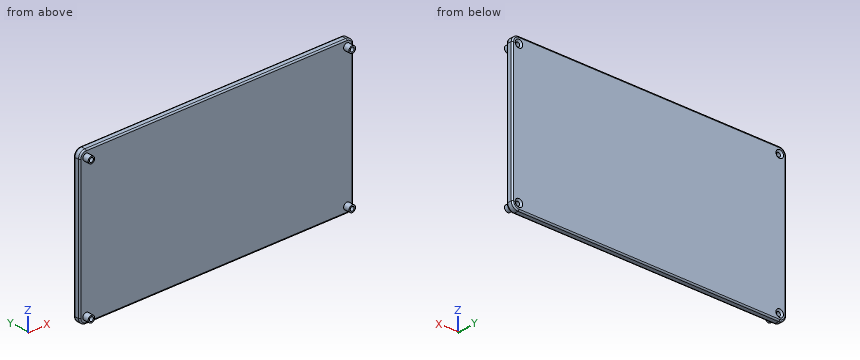
```python
from build123d import *

# Parameters (mm, degrees)
SKETCH1_W                                         = 210
SKETCH1_H                                         = 113
BOSS_EXTRUDE1_DEPTH                               = 5
FILLET1_R                                         = 5
FILLET2_R                                         = 1
CSK_FOR_4_FLAT_HEAD_MACHINE_SCREW_100_D           = 2.9464
CSK_FOR_4_FLAT_HEAD_MACHINE_SCREW_100_CSINK_D     = 5.715
CSK_FOR_4_FLAT_HEAD_MACHINE_SCREW_100_CSINK_ANGLE = 100
SKETCH8_R                                         = 2.4732
BOSS_EXTRUDE2_DEPTH                               = 4.525
SKETCH10_R                                        = 1.525
CUT_EXTRUDE1_DEPTH                                = 1
CUT_EXTRUDE1_DEPTH_BACK                           = 10.525
SKETCH11_R                                        = 2.525
BOSS_EXTRUDE3_DEPTH                               = 4.525
SKETCH14_R                                        = 1.525
CUT_EXTRUDE2_DEPTH                                = 10.5250001
SKETCH15_R                                        = 2.525
BOSS_EXTRUDE6_DEPTH                               = 4.525
SKETCH16_R                                        = 1.525
CUT_EXTRUDE3_DEPTH                                = 10.5250001
SKETCH17_R                                        = 2.525
BOSS_EXTRUDE7_DEPTH                               = 4.525
SKETCH18_R                                        = 1.525
CUT_EXTRUDE4_DEPTH                                = 10.5250001


with BuildPart() as part:
    # Sketch1 → Boss-Extrude1 (new body)
    with BuildSketch(Plane(origin=(0, 0, 0), x_dir=(1, 0, 0), z_dir=(0, 1, 0))):
        Rectangle(SKETCH1_W, SKETCH1_H)
    extrude(amount=BOSS_EXTRUDE1_DEPTH)

    # Fillet1
    fillet1_edges = [part.edges().sort_by_distance(p)[0] for p in [
        (105, 2.5, 56.5),
        (-105, 2.5, 56.5),
        (-105, 2.5, -56.5),
        (105, 2.5, -56.5),
    ]]
    fillet(fillet1_edges, radius=FILLET1_R)

    # Fillet2
    fillet2_edges = [part.edges().sort_by_distance(p)[0] for p in [
        (-105, 0, 0),
        (-105, 5, 0),
        (105, 0, 0),
        (0, 0, 56.5),
        (0, 0, -56.5),
        (103.535533906, 0, -55.035533906),
        (103.535533906, 0, 55.035533906),
        (-103.535533906, 0, 55.035533906),
        (-103.535533906, 0, -55.035533906),
        (0, 5, -56.5),
        (105, 5, 0),
        (0, 5, 56.5),
        (103.535533906, 5, -55.035533906),
        (103.535533906, 5, 55.035533906),
        (-103.535533906, 5, 55.035533906),
        (-103.535533906, 5, -55.035533906),
    ]]
    fillet(fillet2_edges, radius=FILLET2_R)

    # CSK for #4 Flat Head Machine Screw (100)1 (through all)
    with Locations(Plane(origin=(0, 5, 0), x_dir=(1, 0, 0), z_dir=(0, 1, 0))):
        with Locations((-100, -51.5), (100, 51.5), (100, -51.5), (-100, 51.5)):
            CounterSinkHole(CSK_FOR_4_FLAT_HEAD_MACHINE_SCREW_100_D / 2, CSK_FOR_4_FLAT_HEAD_MACHINE_SCREW_100_CSINK_D / 2, counter_sink_angle=CSK_FOR_4_FLAT_HEAD_MACHINE_SCREW_100_CSINK_ANGLE)

    # Sketch8 → Boss-Extrude2 (add)
    with BuildSketch(Plane.XZ):
        with Locations((-100, 51.5)):
            Circle(SKETCH8_R)
    extrude(amount=BOSS_EXTRUDE2_DEPTH)

    # Sketch10 → Cut-Extrude1 (cut, two sides)
    with BuildSketch(Plane.XZ.offset(4.525)) as cut_extrude1_sk:
        with Locations((-100, 51.5)):
            Circle(SKETCH10_R)
    extrude(amount=CUT_EXTRUDE1_DEPTH, mode=Mode.SUBTRACT)
    extrude(cut_extrude1_sk.sketch, amount=-CUT_EXTRUDE1_DEPTH_BACK, mode=Mode.SUBTRACT)

    # Sketch11 → Boss-Extrude3 (add)
    with BuildSketch(Plane.XZ):
        with Locations((-100, -51.5)):
            Circle(SKETCH11_R)
    extrude(amount=BOSS_EXTRUDE3_DEPTH)

    # Sketch14 → Cut-Extrude2 (cut, through all)
    with BuildSketch(Plane.XZ.offset(4.525)):
        with Locations((-100, -51.5)):
            Circle(SKETCH14_R)
    extrude(amount=-CUT_EXTRUDE2_DEPTH, mode=Mode.SUBTRACT)

    # Sketch15 → Boss-Extrude6 (add)
    with BuildSketch(Plane.XZ):
        with Locations((100, 51.5)):
            Circle(SKETCH15_R)
    extrude(amount=BOSS_EXTRUDE6_DEPTH)

    # Sketch16 → Cut-Extrude3 (cut, through all)
    with BuildSketch(Plane.XZ.offset(4.525)):
        with Locations((100, 51.5)):
            Circle(SKETCH16_R)
    extrude(amount=-CUT_EXTRUDE3_DEPTH, mode=Mode.SUBTRACT)

    # Sketch17 → Boss-Extrude7 (add)
    with BuildSketch(Plane.XZ):
        with Locations((100, -51.5)):
            Circle(SKETCH17_R)
    extrude(amount=BOSS_EXTRUDE7_DEPTH)

    # Sketch18 → Cut-Extrude4 (cut, through all)
    with BuildSketch(Plane.XZ.offset(4.525)):
        with Locations((100, -51.5)):
            Circle(SKETCH18_R)
    extrude(amount=-CUT_EXTRUDE4_DEPTH, mode=Mode.SUBTRACT)


solid = part.part
```
Source: CAD feature listing. Evaluate the final solid. Frame: model axes, mm. Give positions to 0.01 mm unless a question says otherwise; leave off trailing zeros. Write each loop counter-clockwise with the first axis right and the second up, starting at its lowest first coordinate (ties: lowest second). Pieces come first, ordered by that corner, then holes.
1. Section query A-A (y = -2.5). Return the cut outline in (x, z) (3 decimals), then the cut area to 3 significant figures.
2. First-contact query: pin 1 (5 mm diameter, centred on x = 100, z = -51.5, fed in from +Y); pin 2 (3.5 mm diameter, centred on x = -100, z = 51.5, fed in from -Y) (3 decimals). Flat tips, straight axial feed; report the tip coordinate or a pass-through.
3. Section query C-C (x = 42). Return the cut outline in (y, z), then the cut area to 3 significant figures.
4. Material intervals for line 1 along X through (y, z) = (1.5, 51.5) (3 decimals); line 2 along Z through (x, y) = (100, -1.5) (3 decimals); line 3 along X through (y, z) = (3, -51), sorted ascending.
5. Section query B-B (z = -36). Return the cut outline in (x, y), then the cut area to 3 significant figures.
Output values:
1. outline: circle Ø5.05 at (-100, -51.5); circle Ø4.946 at (-100, 51.5); circle Ø5.05 at (100, -51.5); circle Ø5.05 at (100, 51.5); hole circle Ø3.05 at (-100, -51.5); hole circle Ø3.05 at (-100, 51.5); hole circle Ø3.05 at (100, -51.5); hole circle Ø3.05 at (100, 51.5)
1. area: 50.1 mm2
2. pin 1: stops at y = 4.7
2. pin 2: stops at y = -4.525
3. outline: (0, -55.5) arc R1 ccw to (1, -56.5) - (4, -56.5) arc R1 ccw to (5, -55.5) - (5, 55.5) arc R1 ccw to (4, 56.5) - (1, 56.5) arc R1 ccw to (0, 55.5) - close
3. area: 564 mm2
4. line 1: x = -105 to -101.525, -98.475 to 98.475, 101.525 to 105
4. line 2: z = -54.025 to -53.025, -49.975 to -48.975, 48.975 to 49.975, 53.025 to 54.025
4. line 3: x = -105 to -101.44, -98.56 to 98.56, 101.44 to 105
5. outline: (-105, 1) arc R1 ccw to (-104, 0) - (104, 0) arc R1 ccw to (105, 1) - (105, 4) arc R1 ccw to (104, 5) - (-104, 5) arc R1 ccw to (-105, 4) - close
5. area: 1,050 mm2
